Design review of the part built by this model. Coordinates are the model's own, in mm. Give positions to 0.01 mm unless a question says otherwise; leave off trailing zeros. Loops run counter-clockwise (first coordinate to the right, second up) from the corner with the lowest first, then second, coordinate; pieces in that order, holes last.
from build123d import *

# Parameters (mm, degrees)
SKETCH2_R      = 4.8895
SKETCH2_R_2    = 1.7859375
EXTRUDE1_DEPTH = 2.38125


with BuildPart() as part:
    # Sketch2 → Extrude1 (new body)
    with BuildSketch(Plane.ZY):
        with BuildLine():
            Line((7.9375, -7.62), (3.527817924, -7.62))
            ThreePointArc((3.527817924, -7.62), (0, -6.35635), (-3.527817924, -7.62))
            Line((-3.527817924, -7.62), (-7.9375, -7.62))
            ThreePointArc((-7.9375, -7.62), (-10.18256403, -6.69006403), (-11.1125, -4.445))
            Line((-11.1125, -4.445), (-11.1125, 4.445))
            ThreePointArc((-11.1125, 4.445), (-10.18256403, 6.69006403), (-7.9375, 7.62))
            Line((-7.9375, 7.62), (7.9375, 7.62))
            ThreePointArc((7.9375, 7.62), (10.18256403, 6.69006403), (11.1125, 4.445))
            Line((11.1125, 4.445), (11.1125, -4.445))
            ThreePointArc((11.1125, -4.445), (10.18256403, -6.69006403), (7.9375, -7.62))
        make_face()
        Circle(SKETCH2_R, mode=Mode.SUBTRACT)
        with Locations((-7.14375, 4.7625)):
            Circle(SKETCH2_R_2, mode=Mode.SUBTRACT)
        with Locations((7.14375, -4.7625)):
            Circle(SKETCH2_R_2, mode=Mode.SUBTRACT)
    extrude(amount=-EXTRUDE1_DEPTH)


solid = part.part
Q1. Draft analysis for pull direction Y (two halves, no side actions). For faces 1 (the face through (1.174, -6.357, 0.054)), 2 (the face through (1.17, 3.18, -6.32)), 3 (the face through (1, 7.62, 0)), state which applies: pulls with the +Y half, pulls with the -Y half, needs draft (parallel to the pull), parting line crosses it, or undercut.
Results:
face 1: pulls with the -Y half
face 2: undercut
face 3: pulls with the +Y half
Q2. Take a section at D-D (y = -3.25). Give the boundary of the cut face in (x, z).
Results:
outline: (0, -11.11) - (2.38, -11.11) - (2.38, -3.65) - (0, -3.65) - close; (0, 3.65) - (2.38, 3.65) - (2.38, 6.19) - (0, 6.19) - close; (0, 8.09) - (2.38, 8.09) - (2.38, 11.11) - (0, 11.11) - close
Q3. Take a section at C-C (x = 1.15). Give the number of separate pieces and of enclosed holes in the cut face, plus the area to 3 significant figures.
Results:
separate pieces: 1
enclosed holes: 3
area: 229 mm2
Q4. Take a section at B-B (z = 0). Give the boundary of the cut face in (x, y).
Results:
outline: (0, -6.36) - (2.38, -6.36) - (2.38, -4.89) - (0, -4.89) - close; (0, 4.89) - (2.38, 4.89) - (2.38, 7.62) - (0, 7.62) - close
Q5. Take a section at A-A (y = 0). Give the boundary of the cut face in (x, z), plus the area to 3 significant figures.
Results:
outline: (0, -11.11) - (2.38, -11.11) - (2.38, -4.89) - (0, -4.89) - close; (0, 4.89) - (2.38, 4.89) - (2.38, 11.11) - (0, 11.11) - close
area: 29.6 mm2
Q6. Wall thickness on line 1 (Z direction, x = 0.2, y = 3.5); line 2 (Y direction, x = 0.6, z = -3.75); line 3 (Y direction, x = 0.35, z = -6): over which ranges is each line inside the solid? List them lowest first.
Results:
line 1: z = -11.11 to -8.41, -5.88 to -3.41, 3.41 to 11.11
line 2: y = -7.62 to -3.14, 3.14 to 7.62
line 3: y = -7.62 to 3.39, 6.13 to 7.62
Q7. Insertion check: pin 1 (9 mm diameter, centred on y = 0, z = 0, fed in from +X). The pin has a flat end and moves straight along its axis. Give the tip position at first contact, or say it passes through.
Results:
pin 1: passes through
